Study the drawing (mm; zero at the part's minimum x, y, z) and answer. A direction names the side the tool comes from. Round coordinates to 2 decimals unless told otherwise and drop trailing zeros. Order: outer loops, then holes, each group sorted by start corner. A loop starts at its lowest first (then second) coordinate and runs counter-clockwise, first axis right, second up. Notation, with made-up numbers: (18.25, 13) - (44.25, 13) arc R25 ccw to (44.25, 26) - close; hole circle Ø5 at (48, -26). An arc over 180 degrees is marked (long way). Put each result on its own line as item: value.
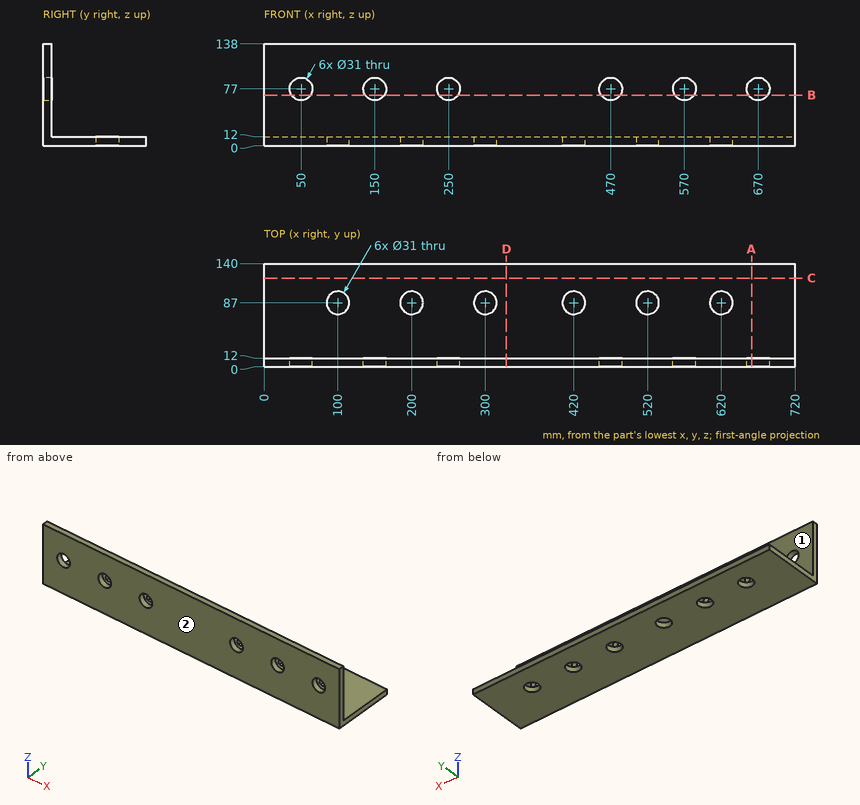
1) A cutting plane is placed at B-B on z = 68.5. Write down the section's boundary in (x, y).
Findings below:
outline: (0, 0) - (37.04, 0) - (37.04, 12) - (0, 12) - close; (62.96, 0) - (137.04, 0) - (137.04, 12) - (62.96, 12) - close; (162.96, 0) - (237.04, 0) - (237.04, 12) - (162.96, 12) - close; (262.96, 0) - (457.04, 0) - (457.04, 12) - (262.96, 12) - close; (482.96, 0) - (557.04, 0) - (557.04, 12) - (482.96, 12) - close; (582.96, 0) - (657.04, 0) - (657.04, 12) - (582.96, 12) - close; (682.96, 0) - (720, 0) - (720, 12) - (682.96, 12) - close
2) A cutting plane is placed at D-D on x = 328.5. Write down the section's boundary in (y, z), then the cut area to 3 significant figures.
Findings below:
outline: (0, 0) - (140, 0) - (140, 12) - (12, 12) - (12, 138) - (0, 138) - close
area: 3,190 mm2
3) For the marked faces 1 and 2, determine the directions among +Z, -Z, +X, -X, +Y, -Y from which every point of the face is accessible in a straight line to the end or side of a thin tool.
Findings below:
face 1: +Z, +X, -X, +Y
face 2: +Z, -Z, +X, -X, -Y
4) Given pin 1 Ø3 at (x, y) = (421.5, 71) entering from +Z; pin 2 Ø5 at (x, z) = (374, 25.5) entering from +Y, each flat-ended and moving along its own axis, determine where each tip first touches the part or whether it passes through.
Findings below:
pin 1: stops at z = 12
pin 2: stops at y = 12
5) A cutting plane is placed at C-C on y = 120.5. Write down the section's boundary in (x, z), then the cut area to 3 significant figures.
Findings below:
outline: (0, 0) - (720, 0) - (720, 12) - (0, 12) - close
area: 8,640 mm2
6) A cutting plane is placed at A-A on x = 661. Write down the section's boundary in (y, z), then the cut area to 3 significant figures.
Findings below:
outline: (0, 0) - (140, 0) - (140, 12) - (12, 12) - (12, 64.38) - (0, 64.38) - close; (0, 89.62) - (12, 89.62) - (12, 138) - (0, 138) - close
area: 2,890 mm2
7) Straight lines are drawn through the part: L1, parallel to Y at x = 659.5, z = 130.5; L2, parallel to Y at x = 92.5, z = 6. For each, find the intervals that lie inside material, in ascending order. Write a range as from..to.
Findings below:
L1: y = 0..12
L2: y = 0..73.44, 100.56..140
